Geometry: final body of the model. Coordinates: model frame, mm. Face numbers are marked on the shaded views. A direction names the side the tool comes from. Round coordinates to 2 decimals unless told otherwise and drop trailing zeros. Write each loop counter-clockwise with the first axis right and the second up, starting at its lowest first coordinate (ties: lowest second). Pieces come first, ordered by that corner, then holes. Notation, with made-up numbers: M -31,80 L 9,80 A30 ccw 9,103 Z; hole C -37.5,20 d9. An arc over 180 degrees is marked long. Use one line per item in the form item = value. Start each with the question number.
Item 1: Section query B-B (x = -7.5). Return loops of the section in (y, z), and give its area (3 significant figures).
Item 2: Pin query (flat end, axial travel): pin 1 Ø3 at (x, z) = (-7, -14.5) entering from +Y; pin 2 Ø9 at (x, z) = (10.5, -5.5) entering from +Y. Return the tip coordinate at first contact, or that it passes through.
Item 3: Reachability of the marked faces 1 and 2 from +Z, -Z, +X, -X, +Y, -Y: full face, straight path, thin tool, end or side. Return the list, or none.
Item 4: Section query A-A (y = 28.5). Return loops of the section in (x, z), and give its area (3 significant figures).
Item 5: Ray query, probe 1 along Z at (x, y) = (25, 25.5); probe 2 along Y at (x, z) = (-15, -13.5); probe 3 along Y at (x, z) = (14, 20.5). Return the intervals inside material, ascending.
Item 6: Section query C-C (z = -4). Return loops of the section in (x, y).
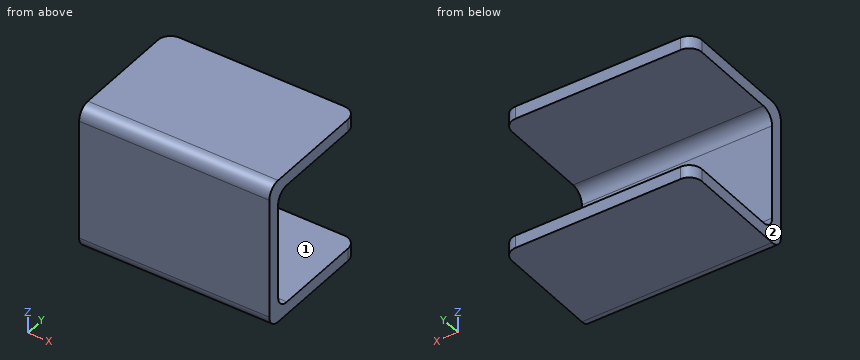
from build123d import *

# Parameters (mm, degrees)
AUFSATZ_LINEAR_AUSTRAGEN1_DEPTH = 30
VERRUNDUNG1_R                   = 4
VERRUNDUNG2_R                   = 4
VERRUNDUNG3_R                   = 4
VERRUNDUNG4_R                   = 4
VERRUNDUNG5_R                   = 4
VERRUNDUNG6_R                   = 4
VERRUNDUNG7_R                   = 4


with BuildPart() as part:
    # Skizze1 → Aufsatz-Linear austragen1 (new, symmetric)
    with BuildSketch(Plane(origin=(0, 0, 0), x_dir=(0, 0, -1), z_dir=(1, 0, 0))):
        Polygon((-23, 40), (-19, 40), (-19, 4), (19, 4), (19, 40), (23, 40), (23, 0), (-23, 0), align=None)
    extrude(amount=AUFSATZ_LINEAR_AUSTRAGEN1_DEPTH, both=True)

    # Verrundung1
    verrundung1_edges = [part.edges().sort_by_distance(p)[0] for p in [
        (0, 0, -23),
    ]]
    fillet(verrundung1_edges, radius=VERRUNDUNG1_R)

    # Verrundung2
    verrundung2_edges = [part.edges().sort_by_distance(p)[0] for p in [
        (0, 0, 23),
    ]]
    fillet(verrundung2_edges, radius=VERRUNDUNG2_R)

    # Verrundung3
    verrundung3_edges = [part.edges().sort_by_distance(p)[0] for p in [
        (-30, 40, -21),
    ]]
    fillet(verrundung3_edges, radius=VERRUNDUNG3_R)

    # Verrundung4
    verrundung4_edges = [part.edges().sort_by_distance(p)[0] for p in [
        (30, 40, -21),
    ]]
    fillet(verrundung4_edges, radius=VERRUNDUNG4_R)

    # Verrundung5
    verrundung5_edges = [part.edges().sort_by_distance(p)[0] for p in [
        (-30, 40, 21),
        (30, 40, 21),
    ]]
    fillet(verrundung5_edges, radius=VERRUNDUNG5_R)

    # Verrundung6
    verrundung6_edges = [part.edges().sort_by_distance(p)[0] for p in [
        (0, 4, 19),
    ]]
    fillet(verrundung6_edges, radius=VERRUNDUNG6_R)

    # Verrundung7
    verrundung7_edges = [part.edges().sort_by_distance(p)[0] for p in [
        (0, 4, -19),
    ]]
    fillet(verrundung7_edges, radius=VERRUNDUNG7_R)


solid = part.part
Working result:
q1.outline = M 0,-19 A4 ccw 4,-23 L 40,-23 L 40,-19 L 8,-19 A4 cw 4,-15 L 4,15 A4 cw 8,19 L 40,19 L 40,23 L 4,23 A4 ccw 0,19 Z
q1.area = 472 mm²
q2.pin_1 = 4.13
q2.pin_2 = 4
q3.face_1 = +X, -X, +Y
q3.face_2 = +Z, -Z, -X, +Y, -Y
q4.outline = M -30,-23 L 30,-23 L 30,-19 L -30,-19 Z; M -30,19 L 30,19 L 30,23 L -30,23 Z
q4.area = 480 mm²
q5.probe_1 = -23 to -19, 19 to 23
q5.probe_2 = 0 to 4
q5.probe_3 = 0.29 to 40
q6.outline = M -30,0 L 30,0 L 30,4 L -30,4 Z
